Part model, mm, in its own coordinate system. Coordinates: 2 decimals unless noted, no trailing zeros. Write each loop counter-clockwise with the first axis right and the second up, starting at its lowest first coordinate (ties: lowest second). Pieces come first, ordered by that corner, then holes. Notation, with made-up numbers: M 82,46.25 L 120,46.25 A30 cw 120,79.25 Z; hole C 28,-0.5 d2. An arc over 180 degrees is marked long. Use a Markdown table: item, result. Add a question column.
Q1. Mould opens along Z. For faces 1 (the flat face through (0, 1, 1)), 2 (the cylindrical face through (1.97, -62.78, 13.94)), 3 (the cylindrical face through (1.97, -26.92, -47.92)) say: released by +Z, released by -Z, zero draft, split by the parting line, or undercut.
Q2. Slice it at D-D on y = 34.5. Write the cut outline in (x, z), then the cut area to 3 significant figures.
Q3. Slice it at B-B on x = 2.45. Count the separate pieces of the cut face and the enclosed holes in it, then the cut area to 3 significant figures.
Q4. Wall check: L1, parallel to Y at x = 0.9, z = 0; L2, parallel to Y at x = 1.35, z = -40; L3, parallel to Y at x = 0.5, z = -46. Give the ranges that are in metal, low to high. Write a range as from..to.
Q5. Pin check, flat tips, straight feed: pin 1 Ø1.5 at (y, z) = (-29.88, -51.75) entering from +X; pin 2 Ø2 at (x, z) = (1.5, -37.5) entering from +Y; pin 3 Ø1.5 at (x, z) = (3.5, 21) entering from -Y. Stop position of each tip, or through.
Q6. Slice it at A-A on y = -25. Write the cut outline in (x, z), then the cut area to 3 significant figures.
Q7. Slice it at C-C on z = -23. Write the cut outline in (x, y).
from build123d import *

# Parameters (mm, degrees)
SKETCH1_R           = 64.308589671
SKETCH1_R_2         = 1.25
SKETCH1_R_3         = 5
BOSS_EXTRUDE2_DEPTH = 4


with BuildPart() as part:
    # Sketch1 → Boss-Extrude2 (new body)
    with BuildSketch(Plane(origin=(0, 0, 0), x_dir=(0, 0, -1), z_dir=(1, 0, 0))):
        Circle(SKETCH1_R)
        with Locations((51.745017876, -29.875)):
            Circle(SKETCH1_R_2, mode=Mode.SUBTRACT)
        with Locations((0, 50)):
            Circle(SKETCH1_R_3, mode=Mode.SUBTRACT)
        with Locations((48.176270189, -16.556252313)):
            Circle(SKETCH1_R_2, mode=Mode.SUBTRACT)
        with Locations((43.301270189, -25)):
            Circle(SKETCH1_R_3, mode=Mode.SUBTRACT)
        with Locations((0, 59.75)):
            Circle(SKETCH1_R_2, mode=Mode.SUBTRACT)
        with Locations((9.75, 50)):
            Circle(SKETCH1_R_2, mode=Mode.SUBTRACT)
        with Locations((0, 40.25)):
            Circle(SKETCH1_R_2, mode=Mode.SUBTRACT)
        with Locations((-9.75, 50)):
            Circle(SKETCH1_R_2, mode=Mode.SUBTRACT)
        with Locations((38.426270189, -33.443747687)):
            Circle(SKETCH1_R_2, mode=Mode.SUBTRACT)
        with Locations((34.857522502, -20.125)):
            Circle(SKETCH1_R_2, mode=Mode.SUBTRACT)
        with Locations((-51.745017876, -29.875)):
            Circle(SKETCH1_R_2, mode=Mode.SUBTRACT)
        with Locations((-38.426270189, -33.443747687)):
            Circle(SKETCH1_R_2, mode=Mode.SUBTRACT)
        with Locations((-43.301270189, -25)):
            Circle(SKETCH1_R_3, mode=Mode.SUBTRACT)
        with Locations((-48.176270189, -16.556252313)):
            Circle(SKETCH1_R_2, mode=Mode.SUBTRACT)
        with Locations((-34.857522502, -20.125)):
            Circle(SKETCH1_R_2, mode=Mode.SUBTRACT)
    extrude(amount=BOSS_EXTRUDE2_DEPTH)


solid = part.part
Recorded:
| question | item | result |
|---|---|---|
| 1 | face 1 | zero draft |
| 1 | face 2 | split by the parting line |
| 1 | face 3 | undercut |
| 2 | outline | M 0,-54.27 L 4,-54.27 L 4,54.27 L 0,54.27 Z |
| 2 | area | 434 mm² |
| 3 | separate pieces | 1 |
| 3 | enclosed holes | 15 |
| 3 | area | 12,700 mm² |
| 4 | L1 | -64.31..39, 41.5..45, 55..58.5, 61..64.31 |
| 4 | L2 | -50.35..-28.76, -21.24..50.35 |
| 4 | L3 | -44.94..-29.21, -20.79..44.94 |
| 5 | pin 1 | through |
| 5 | pin 2 | y = 52.95 |
| 5 | pin 3 | y = -61.04 |
| 6 | outline | M 0,-59.25 L 4,-59.25 L 4,-48.3 L 0,-48.3 Z; M 0,-38.3 L 4,-38.3 L 4,38.3 L 0,38.3 Z; M 0,48.3 L 4,48.3 L 4,59.25 L 0,59.25 Z |
| 6 | area | 394 mm² |
| 7 | outline | M 0,-60.05 L 4,-60.05 L 4,60.05 L 0,60.05 Z |
